from build123d import *

# Parameters (mm, degrees)
SALIENTE_EXTRUIR1_DEPTH = 1
SALIENTE_EXTRUIR2_DEPTH = 27.5
REDONDEO1_R             = 2
CORTAR_EXTRUIR1_DEPTH   = 3


with BuildPart() as part:
    # Croquis1 → Saliente-Extruir1 (new body)
    with BuildSketch(Plane(origin=(0, 0, 0), x_dir=(1, 0, 0), z_dir=(0, 1, 0))):
        with BuildLine():
            Line((-115.079714212, -8.823380035), (-63.118189984, -98.823380035))
            ThreePointArc((-63.118189984, -98.823380035), (-57.627808928, -104.313761092), (-50.127808928, -106.323380035))
            Line((-50.127808928, -106.323380035), (-41.46755489, -106.323380035))
            Line((-41.46755489, -106.323380035), (71.115747602, 88.676619965))
            Line((71.115747602, 88.676619965), (66.785620583, 96.176619965))
            ThreePointArc((66.785620583, 96.176619965), (66.062943429, 97.308157543), (65.241980727, 98.37054156))
            Line((65.241980727, 98.37054156), (65.207007249, 98.329234857))
            Line((65.207007249, 98.329234857), (63.414251951, 96.211835777))
            ThreePointArc((63.414251951, 96.211835777), (57.625242859, 94.922266282), (55.376892454, 100.410484227))
            Line((55.376892454, 100.410484227), (56.341107438, 103.402342517))
            Line((56.341107438, 103.402342517), (56.358401529, 103.456004274))
            ThreePointArc((56.358401529, 103.456004274), (55.08155896, 103.621364269), (53.795239526, 103.676619965))
            Line((53.795239526, 103.676619965), (-50.127808928, 103.676619965))
            ThreePointArc((-50.127808928, 103.676619965), (-57.627808928, 101.667001022), (-63.118189984, 96.176619965))
            Line((-63.118189984, 96.176619965), (-115.079714212, 6.176619965))
            ThreePointArc((-115.079714212, 6.176619965), (-117.089333155, -1.323380035), (-115.079714212, -8.823380035))
        make_face()
    extrude(amount=SALIENTE_EXTRUIR1_DEPTH)

    # Croquis2 → Saliente-Extruir2 (add)
    with BuildSketch(Plane.XZ):
        Polygon((70.538397333, -89.676619965), (71.115747602, -88.676619965), (-41.46755489, 106.323380035), (-42.622255428, 106.323380035), align=None)
    extrude(amount=SALIENTE_EXTRUIR2_DEPTH)

    # Redondeo1
    redondeo1_edges = [part.edges().sort_by_distance(p)[0] for p in [
        (13.958070952, 0, 8.323380035),
        (14.824096356, 1, 8.823380035),
    ]]
    fillet(redondeo1_edges, radius=REDONDEO1_R)

    # Croquis3 → Cortar-Extruir1 (cut)
    with BuildSketch(Plane(origin=(14.938707896, 0, 8.624867025), x_dir=(0.49999999999999983, 0, -0.8660254037844387), z_dir=(0.8660254037844387, 0, 0.49999999999999983))):
        with BuildLine():
            Line((-117.14265259, 2.577906999), (-128.509159891, -12.943048078))
            Line((-128.509159891, -12.943048078), (-113.226187721, -43.828381759))
            Line((-113.226187721, -43.828381759), (121.292947467, -43.828381759))
            Line((121.292947467, -43.828381759), (140.229409901, -2.708549898))
            Line((140.229409901, -2.708549898), (116.684206431, 2.577906999))
            add(Edge.make_bspline(
                [(86.373317299, -27.422093001), (116.684206431, -27.422093001), (116.684206431, 2.577906999)],
                knots=[1.570796327, 1.570796327, 1.570796327, 3.141592654, 3.141592654, 3.141592654], degree=2, weights=[1, 0.707106781, 1]))
            Line((86.373317299, -27.422093001), (-86.831763458, -27.422093001))
            add(Edge.make_bspline(
                [(-117.14265259, 2.577906999), (-117.14265259, -27.422093001), (-86.831763458, -27.422093001)],
                knots=[3.141592654, 3.141592654, 3.141592654, 4.71238898, 4.71238898, 4.71238898], degree=2, weights=[1, 0.707106781, 1]))
        make_face()
    extrude(amount=-CORTAR_EXTRUIR1_DEPTH, mode=Mode.SUBTRACT)


solid = part.part
Source: CAD feature listing. Evaluate the final solid. Frame: model axes, mm. A direction names the side the tool comes from. Round coordinates to 2 decimals unless told otherwise and drop trailing zeros. Write each loop counter-clockwise with the first axis right and the second up, starting at its lowest first coordinate (ties: lowest second). Pieces come first, ordered by that corner, then holes. Notation, with made-up numbers: M -24.75,30.25 L 21.25,30.25 A34 cw 21.25,65.25 Z; hole C -1.5,84.5 d10. An arc over 180 degrees is marked long. One line per item, written item: value. Start each with the question number.
Item 1: Pin query (flat end, axial travel): pin 1 (1.5 mm diameter, centred on y = -12, z = 11, fed in from -X); pin 2 (1.5 mm diameter, centred on y = -3, z = 78.5, fed in from -X); pin 3 (3 mm diameter, centred on x = -24.5, y = -13.5, fed in from +Z). Return the tip coordinate at first contact, or that it passes through.
Item 2: Section query A-A (y = -7.5). Return the cut outline in (x, z), plus the area to 3 significant figures.
Item 3: Mould query, pull axis X, two halves, no side actions, for faces 1 (the cylindrical face through (15.1, 0.43, 7.14)), 2 (the flat face through (-25, 1, -23)), 3 (the cylindrical face through (57.71, 0.49, -94.88)). Classes: pulls with the +X half, pulls with the -X half, needs draft (parallel to the pull), parting line crosses it, or undercut.
Item 4: Set-up query: faces 4 (the flat face through (13.166, -14.533, 9.695)), 5 (the flat face through (-89.463, 0.493, 53.193)). Return all of +Z, -Z, +X, -X, +Y, -Y with unobstructed straight access to the full face (end or side cutting, diameter ignored); none if empty.
Item 5: Ray query, L1, parallel to Y at x = 10, z = -66.5; L2, parallel to X at y = -18.5, z = -75.5; L3, parallel to X at y = -6.5, z = 67. Return the intervals inside material, ascending. Write a range as from..to.
Result set:
1. pin 1: stops at x = 11.98
1. pin 2: stops at x = -26.99
1. pin 3: stops at z = 79.53
2. outline: M -42.62,106.32 L 70.54,-89.68 L 71.12,-88.68 L -41.47,106.32 Z
2. area: 226 mm²
3. face 1: pulls with the +X half
3. face 2: needs draft
3. face 3: undercut
4. face 4: -Z, -X, -Y
4. face 5: +Z, -X, +Y, -Y
5. L1: y = 0..1
5. L2: x = 62.35..63.51
5. L3: x = -19.92..-18.76
